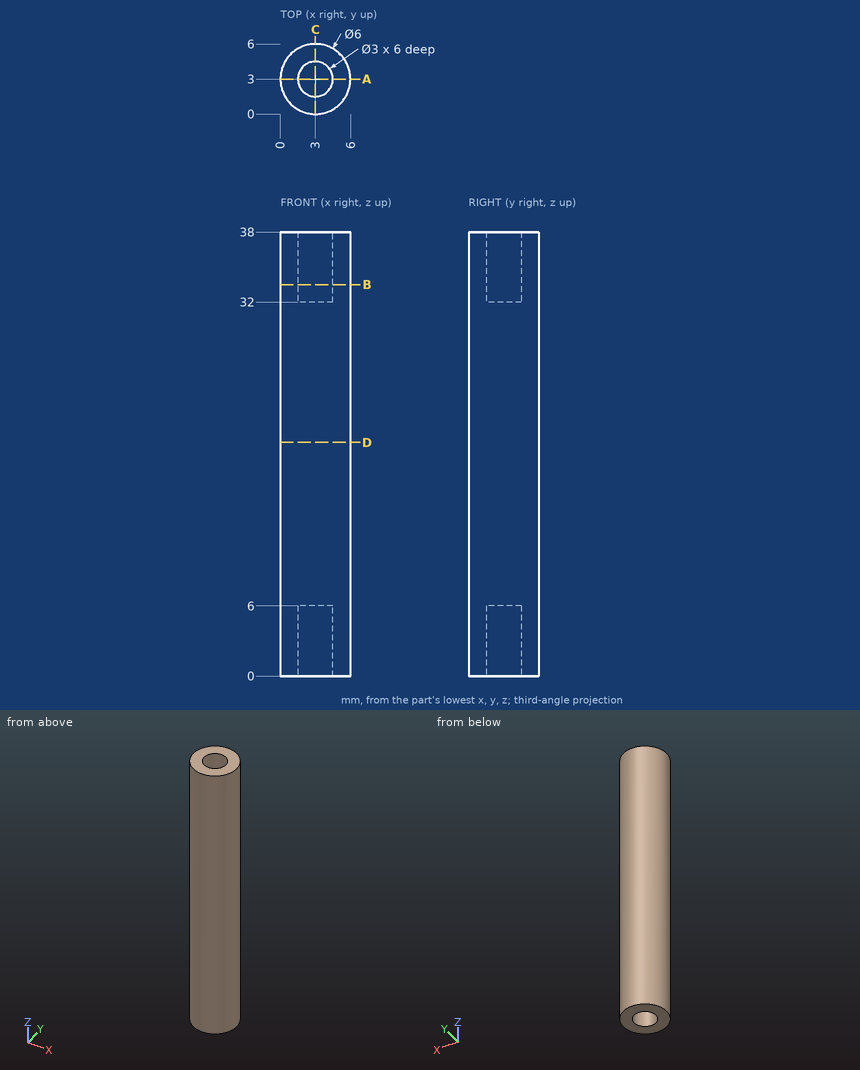
Here's the drawing with two shaded views (mm, measured from the low corner). I have some questions. Coordinates: 2 decimals unless noted, no trailing zeros. Order: outer loops, then holes, each group sorted by start corner. A loop starts at its lowest first (then second) coordinate and runs counter-clockwise, first axis right, second up. Notation, with made-up numbers: (-14.75, 24.5) - (30.25, 24.5) arc R23 ccw to (30.25, 51.5) - close; hole circle Ø1 at (-31.75, 14.5). An arc over 180 degrees is marked (long way). Use CSV: the item, a comma, the result in double quotes. Start each with the question number.
1. Suppose I cut it at B-B on z = 33.5. List the corners of the cut face in (x, y) for me, then the cut area to 3 significant figures.
2. I'm going to push flat-ended pins straight in: pin 1 (2.5 mm diameter, centred on x = 3, y = 3, fed in from -Z); pin 2 (2.5 mm diameter, centred on x = 3.5, y = 3, fed in from +Z). Where does each tip first touch, or does it pass through?
3. Suppose I cut it at D-D on z = 20. List the corners of the cut face in (x, y) for me.
4. Please list where these lines run through material, in increasing order: line 1 (Y direction, x = 3, z = 35.1); line 2 (Z direction, x = 2, y = 3.05); line 3 (Y direction, x = 2.6, z = 34). Write a range as from..to.
5. Suppose I cut it at A-A on y = 3. List the corners of the cut face in (x, z) for me, then the cut area to 3 significant figures.
Output:
1,outline,"circle Ø6 at (3, 3); hole circle Ø3 at (3, 3)"
1,area,"21.2 mm2"
2,pin 1,"stops at z = 6"
2,pin 2,"stops at z = 38"
3,outline,"circle Ø6 at (3, 3)"
4,line 1,"y = 0..1.5, 4.5..6"
4,line 2,"z = 6..32"
4,line 3,"y = 0.03..1.55, 4.45..5.97"
5,outline,"(0, 0) - (1.5, 0) - (1.5, 6) - (4.5, 6) - (4.5, 0) - (6, 0) - (6, 38) - (4.5, 38) - (4.5, 32) - (1.5, 32) - (1.5, 38) - (0, 38) - close"
5,area,"192 mm2"
